Work out the finished part from the listing and answer in its coordinate system (mm). A direction names the side the tool comes from. Round coordinates to 2 decimals unless told otherwise and drop trailing zeros. Loops run counter-clockwise (first coordinate to the right, second up) from the corner with the lowest first, then second, coordinate; pieces in that order, holes last. Notation, with made-up numbers: (72.25, 88) -> (106.25, 88) arc R19 cw to (106.25, 125) -> close; hole circle Ø8 at (36, 78.25). An arc over 180 degrees is marked (long way). Use CSV: the item, a comma, the result in double quotes. Start each with the question number.
from build123d import *

# Parameters (mm, degrees)
F0_W     = 624.14
F0_H     = 366.36
F1_DEPTH = 9.3
F2_W     = 580
F2_H     = 330
F3_DEPTH = 3
F4_W     = 300
F4_H     = 180
F5_DEPTH = 25.4
F6_R     = 15
F7_DEPTH = 15


with BuildPart() as f1:
    # F0 (on Right) → F1 (new body)
    with BuildSketch(Plane.YZ):
        with Locations((-0.668731, 0)):
            Rectangle(F0_W, F0_H)
    extrude(amount=F1_DEPTH)

    # F2 (on face) → F3 (cut)
    with BuildSketch(Plane.YZ.offset(9.3)):
        Rectangle(F2_W, F2_H)
    extrude(amount=-F3_DEPTH, mode=Mode.SUBTRACT)

    # F4 (on Right) → F5 (join)
    with BuildSketch(Plane.YZ):
        Rectangle(F4_W, F4_H)
    extrude(amount=-F5_DEPTH)

    # F6 (on face) → F7 (cut)
    with BuildSketch(Plane(origin=(-25.4, 0, 0), x_dir=(0, -1, 0), z_dir=(-1, 0, 0))):
        Circle(F6_R)
    extrude(amount=-F7_DEPTH, mode=Mode.SUBTRACT)


solid = f1.part
Q1. Section B-B, the plane y = 59 is taken. Write down the section's boundary in (x, z), and give its area (3 significant figures).
Q2. Section A-A, the plane z = 107 is taken. Write down the section's boundary in (x, y).
Q3. Straight lines are drawn through the part: line 1 (Z direction, x = -18.75, y = 0); line 2 (Z direction, x = -12, y = 2); line 3 (X direction, y = -101, z = 46.5). For each, find the intervals that lie inside material, in ascending order. Write a range as from..to.
Q4. Section D-D, the plane z = 0 is taken. Write down the section's boundary in (x, y), and give its area (3 significant figures).
Q5. For a pull along Z with two mould halves and no side action, classify faces 1 (the flat face through (0, -5, 125)), 2 (the flat face through (-13, -2, -90)), 3 (the cylindrical face through (-18.005, 14.985, 0.66)), 4 (the flat face through (-13, -2, 90)) as pulls with the +Z half, pulls with the -Z half, needs draft (parallel to the pull), parting line crosses it, or undercut.
Q6. Which of the six approach directions +Z, -Z, +X, -X, +Y, -Y give full straight-line access (tool end or side, diameter ignored) to faces 5 (the flat face through (-10.4, 0, 0)), 6 (the flat face through (6.3, -4, 2)), 7 (the flat face through (-13, -150, -1)), 8 (the flat face through (-13, 150, -1)), 9 (the flat face through (-25.4, -2, 21))?
Q7. Each of these flat-tipped pins is pushed along its axis until it touches: pin 1 (5 mm diameter, centred on y = -88.5, z = -5.5, fed in from +X); pin 2 (7.5 mm diameter, centred on x = -13.5, y = -53, fed in from +Z); pin 3 (20.5 mm diameter, centred on x = -14, z = 19.5, fed in from +Y). Where does it stop, or does it pass through?
Q8. Section C-C, the plane y = 175 is taken. Write down the section's boundary in (x, z), and give its area (3 significant figures).
Report:
1,outline,"(-25.4, -90) -> (0, -90) -> (0, -183.18) -> (9.3, -183.18) -> (9.3, -165) -> (6.3, -165) -> (6.3, 165) -> (9.3, 165) -> (9.3, 183.18) -> (0, 183.18) -> (0, 90) -> (-25.4, 90) -> close"
1,area,"6,990 mm²"
2,outline,"(0, -312.74) -> (9.3, -312.74) -> (9.3, -290) -> (6.3, -290) -> (6.3, 290) -> (9.3, 290) -> (9.3, 311.4) -> (0, 311.4) -> close"
3,line 1,"z = -90..-15, 15..90"
3,line 2,"z = -90..-14.87, 14.87..90"
3,line 3,"x = -25.4..6.3"
4,outline,"(-25.4, -150) -> (0, -150) -> (0, -312.74) -> (9.3, -312.74) -> (9.3, -290) -> (6.3, -290) -> (6.3, 290) -> (9.3, 290) -> (9.3, 311.4) -> (0, 311.4) -> (0, 150) -> (-25.4, 150) -> (-25.4, 15) -> (-10.4, 15) -> (-10.4, -15) -> (-25.4, -15) -> close"
4,area,"11,200 mm²"
5,face 1,"needs draft"
5,face 2,"pulls with the -Z half"
5,face 3,"undercut"
5,face 4,"pulls with the +Z half"
6,face 5,"-X"
6,face 6,"+X"
6,face 7,"+Z, -Z, -X, -Y"
6,face 8,"+Z, -Z, -X, +Y"
6,face 9,"+Z, -Z, -X, +Y, -Y"
7,pin 1,"stops at x = 6.3"
7,pin 2,"stops at z = 90"
7,pin 3,"stops at y = 150"
8,outline,"(0, -183.18) -> (9.3, -183.18) -> (9.3, -165) -> (6.3, -165) -> (6.3, 165) -> (9.3, 165) -> (9.3, 183.18) -> (0, 183.18) -> close"
8,area,"2,420 mm²"
